```python
from build123d import *

# Parameters (mm, degrees)
F0_R      = 25.4
F1_DEPTH  = 38.1
F2_R      = 38.1
F2_R_2    = 25.4
F3_DEPTH  = 5.08
F4_R      = 38.1
F5_DEPTH  = 5.08
F6_R      = 19.05
F3_FACE_R = 38.1
F7_DEPTH  = 12.7
F8_R      = 19.05
F9_DEPTH  = 12.7
F10_R     = 12.7
F11_DEPTH = 35.561
F12_SIZE  = 1.27


with BuildPart() as f1:
    # F0 (on Right) → F1 (new body)
    with BuildSketch(Plane.YZ):
        Circle(F0_R)
    extrude(amount=F1_DEPTH)

    # F2 (on face) → F3 (join)
    with BuildSketch(Plane.YZ.offset(38.1)):
        Circle(F2_R)
        Circle(F2_R_2, mode=Mode.SUBTRACT)
        Circle(F2_R_2)
    extrude(amount=F3_DEPTH)

    # F4 (on face) → F5 (join)
    with BuildSketch(Plane(origin=(0, 0, 0), x_dir=(0, -1, 0), z_dir=(-1, 0, 0))):
        Circle(F4_R)
    extrude(amount=F5_DEPTH)

    # F6 (on face) + F3_face (on face) → F7 (cut)
    with BuildSketch(Plane(origin=(-5.08, 0, 0), x_dir=(0, -1, 0), z_dir=(-1, 0, 0))):
        Circle(F6_R)
    with BuildSketch(Plane.YZ.offset(43.18)):
        Circle(F3_FACE_R)
    extrude(amount=-F7_DEPTH, dir=(-1, 0, 0), mode=Mode.SUBTRACT)

    # F8 (on face) → F9 (cut)
    with BuildSketch(Plane.YZ.offset(43.18)):
        Circle(F8_R)
    extrude(amount=-F9_DEPTH, mode=Mode.SUBTRACT)

    # F10 (on face) → F11 (cut, through all)
    with BuildSketch(Plane.YZ.offset(30.48)):
        Circle(F10_R)
    extrude(amount=-F11_DEPTH, mode=Mode.SUBTRACT)

    # F12
    f12_edges = [f1.edges().sort_by_distance(p)[0] for p in [
        (0, 38.1, 0),
        (38.1, -38.1, 0),
    ]]
    chamfer(f12_edges, length=F12_SIZE)


solid = f1.part
```
Source: CAD feature listing. Evaluate the final solid. Frame: model axes, mm. A direction names the side the tool comes from. Give positions to 0.01 mm unless a question says otherwise; leave off trailing zeros. Loops run counter-clockwise (first coordinate to the right, second up) from the corner with the lowest first, then second, coordinate; pieces in that order, holes last. Notation, with made-up numbers: (15, 85) -> (38, 85) arc R12 ccw to (38, 98) -> close; hole circle Ø5 at (-34.5, 5). An arc over 180 degrees is marked (long way). Use a Markdown table: item, result. Add a question column.
(1) Ray query, line 1 (X direction, y = 9, z = -25.5); line 2 (Z direction, x = 2.25, y = 0); line 3 (Z direction, x = 22.5, y = 0). Return the intervals inside material, ascending.
(2) Section query A-A (z = 0). Output: boundary loops of the cut face in (x, y).
(3) First-contact query: pin 1 Ø22 at (y, z) = (-11.5, -10) entering from +X; pin 2 Ø23 at (y, z) = (0, 0) entering from -X; pin 3 Ø3 at (x, z) = (28.5, -20) entering from -Y; pin 4 Ø10 at (x, z) = (27.5, -0.5) entering from +Y. Flat tips, straight axial feed; report the tip coordinate or a pass-through.
(4) Access query for faces 4 (the face through (43.18, 7.9, 17.5)), 5 (the face through (36.92, -15.12, -11.59)), 6 (the face through (7.62, -4, -12.4)), 7 (the face through (18.783, -5.506, -24.796)), 8 (the face through (19.21, -2.75, -12.4)). Directions: +Z, -Z, +X, -X, +Y, -Y. A direction counts if a zero-diameter tool reaches every point of the face in a straight line with its end or side. Return the directions, or none.
(5) Section query C-C (x = 36). Output: boundary loops of the cut face in (y, z).
(6) Pull-direction query (Y, two-part tool) for faces 1 (the face through (1.18, 15.12, -11.59)), 2 (the face through (41.248, -30.235, -23.183)), 3 (the face through (-5.08, -7.9, 17.5)); classes: +Y half, -Y half, draft (parallel to the pull), parting line (faces both ways), or undercut.
Checked values:
| question | item | result |
|---|---|---|
| 1 | line 1 | -5.08 to 0, 38.1 to 43.18 |
| 1 | line 2 | -25.4 to -19.05, 19.05 to 25.4 |
| 1 | line 3 | -25.4 to -12.7, 12.7 to 25.4 |
| 2 | outline | (-5.08, -38.1) -> (-1.27, -38.1) -> (0, -36.83) -> (0, -25.4) -> (38.1, -25.4) -> (38.1, -36.83) -> (39.37, -38.1) -> (43.18, -38.1) -> (43.18, -19.05) -> (30.48, -19.05) -> (30.48, -12.7) -> (7.62, -12.7) -> (7.62, -19.05) -> (-5.08, -19.05) -> close; (-5.08, 19.05) -> (7.62, 19.05) -> (7.62, 12.7) -> (30.48, 12.7) -> (30.48, 19.05) -> (43.18, 19.05) -> (43.18, 38.1) -> (39.37, 38.1) -> (38.1, 36.83) -> (38.1, 25.4) -> (0, 25.4) -> (0, 36.83) -> (-1.27, 38.1) -> (-5.08, 38.1) -> close |
| 3 | pin 1 | x = 43.18 |
| 3 | pin 2 | through |
| 3 | pin 3 | y = -17.4 |
| 3 | pin 4 | y = 25.4 |
| 4 | face 4 | +Z, -Z, +X, +Y, -Y |
| 4 | face 5 | +X |
| 4 | face 6 | -X |
| 4 | face 7 | none |
| 4 | face 8 | +X, -X |
| 5 | outline | circle Ø50.8 at (0, 0); hole circle Ø38.1 at (0, 0) |
| 6 | face 1 | undercut |
| 6 | face 2 | parting line |
| 6 | face 3 | draft |
